```python
from build123d import *

# Parameters (mm, degrees)
SKETCH1_W           = 160
SKETCH1_H           = 100
BOSS_EXTRUDE1_DEPTH = 10
SKETCH2_W           = 40
SKETCH2_H           = 20
CUT_EXTRUDE1_DEPTH  = 10
SKETCH3_W           = 6
SKETCH3_H           = 20
BOSS_EXTRUDE2_DEPTH = 10
SKETCH4_W           = 40
SKETCH4_H           = 20
CUT_EXTRUDE2_DEPTH  = 4
SKETCH5_W           = 15
SKETCH5_H           = 4
BOSS_EXTRUDE3_DEPTH = 10
CUT_EXTRUDE3_DEPTH  = 100
SKETCH8_R           = 2.5
SKETCH8_R_2         = 2
CUT_EXTRUDE4_DEPTH  = 97.43650761
SKETCH10_W          = 6
SKETCH10_H          = 20
BOSS_EXTRUDE5_DEPTH = 14
SKETCH11_W          = 20
SKETCH11_H          = 4
BOSS_EXTRUDE6_DEPTH = 10
SKETCH12_R          = 2
CUT_EXTRUDE5_DEPTH  = 10
SKETCH13_R          = 2.5
CUT_EXTRUDE6_DEPTH  = 10
SKETCH14_W          = 10
SKETCH14_H          = 20
CUT_EXTRUDE7_DEPTH  = 10
SKETCH17_R          = 2
CUT_EXTRUDE8_DEPTH  = 10
SKETCH18_R          = 2.4
CUT_EXTRUDE9_DEPTH  = 4
SKETCH15_R          = 13
SKETCH15_R_2        = 3.5
CUT_EXTRUDE10_DEPTH = 10
RIB1_REACH          = 132.292
SKETCH19_WALL_W     = 317.885406234
SKETCH19_WALL_H     = 5


with BuildPart() as part:
    # Sketch1 → Boss-Extrude1 (new body)
    with BuildSketch(Plane(origin=(0, 0, 0), x_dir=(1, 0, 0), z_dir=(0, 1, 0))):
        Rectangle(SKETCH1_W, SKETCH1_H)
    extrude(amount=BOSS_EXTRUDE1_DEPTH)

    # Sketch2 → Cut-Extrude1 (cut)
    with BuildSketch(Plane(origin=(0, 10, 0), x_dir=(1, 0, 0), z_dir=(0, 1, 0))):
        with Locations((60, 20)):
            Rectangle(SKETCH2_W, SKETCH2_H)
        with Locations((60, -20)):
            Rectangle(SKETCH2_W, SKETCH2_H)
    extrude(amount=-CUT_EXTRUDE1_DEPTH, mode=Mode.SUBTRACT)

    # Sketch3 → Boss-Extrude2 (add)
    with BuildSketch(Plane(origin=(0, 10, 0), x_dir=(1, 0, 0), z_dir=(0, 1, 0))):
        with Locations((37, 20)):
            Rectangle(SKETCH3_W, SKETCH3_H)
        with Locations((37, -20)):
            Rectangle(SKETCH3_W, SKETCH3_H)
    extrude(amount=BOSS_EXTRUDE2_DEPTH)

    # Sketch4 → Cut-Extrude2 (cut)
    with BuildSketch(Plane(origin=(0, 10, 0), x_dir=(1, 0, 0), z_dir=(0, 1, 0))):
        with Locations((60, 40)):
            Rectangle(SKETCH4_W, SKETCH4_H)
        with Locations((60, 0)):
            Rectangle(SKETCH4_W, SKETCH4_H)
        with Locations((60, -40)):
            Rectangle(SKETCH4_W, SKETCH4_H)
    extrude(amount=-CUT_EXTRUDE2_DEPTH, mode=Mode.SUBTRACT)

    # Sketch5 → Boss-Extrude3 (add)
    with BuildSketch(Plane(origin=(0, 10, 0), x_dir=(1, 0, 0), z_dir=(0, 1, 0))):
        with Locations((26.5, 28)):
            Rectangle(SKETCH5_W, SKETCH5_H)
        with Locations((26.5, 12)):
            Rectangle(SKETCH5_W, SKETCH5_H)
        with Locations((26.5, -12)):
            Rectangle(SKETCH5_W, SKETCH5_H)
        with Locations((26.5, -28)):
            Rectangle(SKETCH5_W, SKETCH5_H)
    extrude(amount=BOSS_EXTRUDE3_DEPTH)

    # Sketch6 → Cut-Extrude3 (cut)
    with BuildSketch(Plane(origin=(0, 0, -30), x_dir=(-1, 0, 0), z_dir=(0, 0, -1))):
        Polygon((-19, 10), (-34, 20), (-19, 20), align=None)
    extrude(amount=-CUT_EXTRUDE3_DEPTH, mode=Mode.SUBTRACT)

    # Sketch8 → Cut-Extrude4 (cut, through all)
    with BuildSketch(Plane.XZ):
        with Locations(Location((75, 40, 0), (0, 0, 270))):
            Circle(SKETCH8_R)
        with Locations(Location((75, 0, 0), (0, 0, 270))):
            Circle(SKETCH8_R)
        with Locations(Location((75, -40, 0), (0, 0, 270))):
            Circle(SKETCH8_R)
        with Locations(Location((45, 40, 0), (0, 0, 270))):
            Circle(SKETCH8_R_2)
        with Locations(Location((45, 0, 0), (0, 0, 270))):
            Circle(SKETCH8_R_2)
        with Locations(Location((45, -40, 0), (0, 0, 270))):
            Circle(SKETCH8_R_2)
    extrude(amount=-CUT_EXTRUDE4_DEPTH, mode=Mode.SUBTRACT)

    # Sketch10 → Boss-Extrude5 (add)
    with BuildSketch(Plane(origin=(0, 10, 0), x_dir=(1, 0, 0), z_dir=(0, 1, 0))):
        with Locations((37, 40)):
            Rectangle(SKETCH10_W, SKETCH10_H)
        with Locations((37, -40)):
            Rectangle(SKETCH10_W, SKETCH10_H)
        with Locations((37, 0)):
            Rectangle(SKETCH10_W, SKETCH10_H)
    extrude(amount=BOSS_EXTRUDE5_DEPTH)

    # Sketch11 → Boss-Extrude6 (add)
    with BuildSketch(Plane(origin=(40, 0, 0), x_dir=(0, 0, -1), z_dir=(1, 0, 0))):
        with Locations((-40, 22)):
            Rectangle(SKETCH11_W, SKETCH11_H)
        with Locations((0, 22)):
            Rectangle(SKETCH11_W, SKETCH11_H)
        with Locations((40, 22)):
            Rectangle(SKETCH11_W, SKETCH11_H)
    extrude(amount=BOSS_EXTRUDE6_DEPTH)

    # Sketch12 → Cut-Extrude5 (cut)
    with BuildSketch(Plane.XZ.offset(-20)):
        with Locations(Location((45, 40, 0), (0, 0, 270))):
            Circle(SKETCH12_R)
        with Locations(Location((45, 0, 0), (0, 0, 270))):
            Circle(SKETCH12_R)
        with Locations(Location((45, -40, 0), (0, 0, 270))):
            Circle(SKETCH12_R)
    extrude(amount=-CUT_EXTRUDE5_DEPTH, mode=Mode.SUBTRACT)

    # Sketch13 → Cut-Extrude6 (cut)
    with BuildSketch(Plane.ZY.offset(-34)):
        with Locations((-20, 14)):
            Circle(SKETCH13_R)
        with Locations((20, 14)):
            Circle(SKETCH13_R)
    extrude(amount=-CUT_EXTRUDE6_DEPTH, mode=Mode.SUBTRACT)

    # Sketch14 → Cut-Extrude7 (cut)
    with BuildSketch(Plane(origin=(0, 10, 0), x_dir=(1, 0, 0), z_dir=(0, 1, 0))):
        with Locations((-75, 40)):
            Rectangle(SKETCH14_W, SKETCH14_H)
        with Locations((-75, -40)):
            Rectangle(SKETCH14_W, SKETCH14_H)
    extrude(amount=-CUT_EXTRUDE7_DEPTH, mode=Mode.SUBTRACT)

    # Sketch17 → Cut-Extrude8 (cut)
    with BuildSketch(Plane(origin=(0, 10, 0), x_dir=(1, 0, 0), z_dir=(0, 1, 0))):
        with Locations(Location((-62.5, 13.5, 0), (0, 0, 270))):
            Circle(SKETCH17_R)
        with Locations(Location((-62.5, -13.5, 0), (0, 0, 270))):
            Circle(SKETCH17_R)
    extrude(amount=-CUT_EXTRUDE8_DEPTH, mode=Mode.SUBTRACT)

    # Sketch18 → Cut-Extrude9 (cut)
    with BuildSketch(Plane.ZY.offset(70)):
        with Locations((40, 5)):
            Circle(SKETCH18_R)
        with Locations((-40, 5)):
            Circle(SKETCH18_R)
    extrude(amount=-CUT_EXTRUDE9_DEPTH, mode=Mode.SUBTRACT)

    # Sketch15 → Cut-Extrude10 (cut)
    with BuildSketch(Plane(origin=(0, 10, 0), x_dir=(1, 0, 0), z_dir=(0, 1, 0))):
        with Locations(Location((-23, 0, 0), (0, 0, 270))):
            Circle(SKETCH15_R)
        with Locations(Location((-23, 27.5, 0), (0, 0, 270))):
            Circle(SKETCH15_R_2)
        with Locations(Location((-23, -27.5, 0), (0, 0, 270))):
            Circle(SKETCH15_R_2)
    extrude(amount=-CUT_EXTRUDE10_DEPTH, mode=Mode.SUBTRACT)

    # Sketch19 wall → Rib1 (add, up to next)
    with BuildSketch(Plane(origin=(7.25, 17, -50), x_dir=(-0.967424963626, -0.253157934407, 0), z_dir=(-0.253157934407, 0.967424963626, 0)), mode=Mode.PRIVATE) as rib1_sk1:
        with Locations((0, 2.5)):
            Rectangle(SKETCH19_WALL_W, SKETCH19_WALL_H)
    rib1_tool1 = extrude(rib1_sk1.sketch, amount=-RIB1_REACH, mode=Mode.PRIVATE) - part.part
    rib1 = rib1_tool1.solids().sort_by_distance((7.25, 17, -50))[0]
    add(rib1)

    # Mirror2: Rib1 across plane
    add(rib1.mirror(Plane.XY))


solid = part.part
```
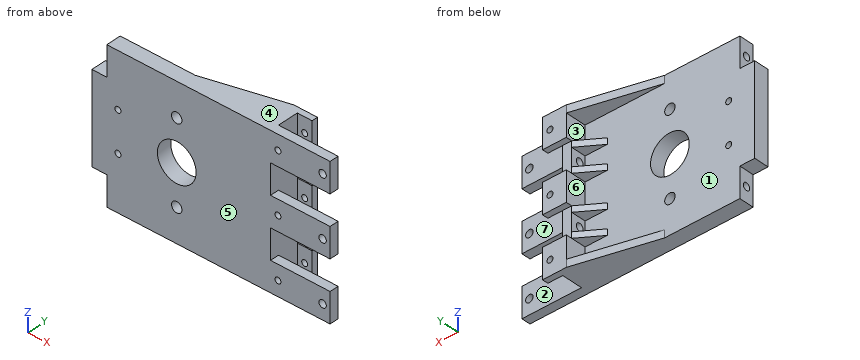
Read the model definition and answer for the solid it produces. Units are mm, in the model's axes. Face numbers are marked on the shaded views. A direction names the side the tool comes from. Give positions to 0.01 mm unless a question says otherwise; leave off trailing zeros. Write each loop counter-clockwise with the first axis right and the second up, starting at its lowest first coordinate (ties: lowest second). Pieces come first, ordered by that corner, then holes. Notation, with made-up numbers: (85, 52) - (134, 52) arc R20 ccw to (134, 86) - close; hole circle Ø11 at (47, -29). An arc over 180 degrees is marked (long way). Write item = value, one per line. Start each with the question number.
Item 1: The mould has two halves that part along Z. Classify the marked faces 1, 2, 3 and 4: +Z half, -Z half, draft (parallel to the pull), parting line (faces both ways), or undercut.
Item 2: Find section C-C (x = 62). Give the vertices of the cut face in (y, z).
Item 3: Each of these flat-tipped pins is pushed along its axis until it touches: P1, Ø4.5, axis at x = 45, z = 0, coming from the -Y side; P2, Ø6, axis at x = 69.5, z = 4.5, coming from the +Y side; P3, Ø8, axis at y = 14, z = -20, coming from the +X side; P4, Ø6.5, axis at x = -62.5, z = 13.5, coming from the +Y side. Where does it stop, or does it pass through?
Item 4: A tool of negligible diameter and unlimited length cuts with its end or side. For the marked faces 5, 6 and 7, from which of +Z, -Z, +X, -X, +Y, -Y can it reach the whole face along a straight path? Write none if from no direction.
Item 5: Find section A-A (x = -23). Give the vertices of the cut face in (y, z), then the cut area to 3 significant figures.
Item 6: Find section B-B (z = 20). Give the vertices of the cut face in (x, y).
Item 7: Find the intervals of material crossed by probe 1 along X at (y, z) = (2.2, 40); probe 2 along Z at (x, y) = (68, 5.5); probe 3 along Z at (x, y) = (-20, 2.75), in increasing order. Write a range as [from, to].
Item 8: Find section D-D (z = 40). Give the vertices of the cut face in (x, y).
Response:
q1.face_1 = undercut
q1.face_2 = draft
q1.face_3 = undercut
q1.face_4 = +Z half
q2.outline = (0, -50) - (6, -50) - (6, -30) - (0, -30) - close; (0, -10) - (6, -10) - (6, 10) - (0, 10) - close; (0, 30) - (6, 30) - (6, 50) - (0, 50) - close
q3.P1 = 0
q3.P2 = 6
q3.P3 = 40
q3.P4 = 10
q4.face_5 = +Z, -Z, +X, -X, -Y
q4.face_6 = -X, +Y
q4.face_7 = +Z, -Z, +X
q5.outline = (0, -50) - (10, -50) - (10, -31) - (0, -31) - close; (0, -24) - (10, -24) - (10, -13) - (0, -13) - close; (0, 13) - (10, 13) - (10, 24) - (0, 24) - close; (0, 31) - (10, 31) - (10, 50) - (0, 50) - close
q5.area = 600 mm²
q6.outline = (-80, 0) - (40, 0) - (40, 11.5) - (34, 11.5) - (34, 10) - (-80, 10) - close; (34, 16.5) - (40, 16.5) - (40, 20) - (34, 20) - close
q7.probe_1 = [-70, 43], [47, 72.5], [77.5, 80]
q7.probe_2 = [-50, -30], [-10, 10], [30, 50]
q7.probe_3 = [-50, -29.3], [-25.7, -12.65], [12.65, 25.7], [29.3, 50]
q8.outline = (-70, 0) - (43, 0) - (43, 6) - (40, 6) - (40, 20) - (43, 20) - (43, 24) - (34, 24) - (34, 10) - (-70, 10) - (-70, 7.4) - (-66, 7.4) - (-66, 2.6) - (-70, 2.6) - close; (47, 0) - (72.5, 0) - (72.5, 6) - (47, 6) - close; (47, 20) - (50, 20) - (50, 24) - (47, 24) - close; (77.5, 0) - (80, 0) - (80, 6) - (77.5, 6) - close
